Model file for the job. Use its own axes, mm. A direction names the side the tool comes from. Round coordinates to 2 decimals unless told otherwise and drop trailing zeros. Loops run counter-clockwise (first coordinate to the right, second up) from the corner with the lowest first, then second, coordinate; pieces in that order, holes last. Notation, with made-up numbers: (86.25, -18.5) -> (114.25, -18.5) arc R24 ccw to (114.25, -2.5) -> close; hole circle Ø9 at (10, 72). An arc over 180 degrees is marked (long way). Use a Markdown table: item, result. Add a question column.
```python
from build123d import *

# Parameters (mm, degrees)
SKETCH1_R           = 38.1
BOSS_EXTRUDE1_DEPTH = 76.2
SKETCH2_W           = 63.5
SKETCH2_H           = 42.121134838
BOSS_EXTRUDE2_DEPTH = 63.5
SKETCH3_W           = 25.4
SKETCH3_H           = 42.121134838
CUT_EXTRUDE1_DEPTH  = 63.5
FILLET1_R           = 25.4
SKETCH5_R           = 25.4
CUT_EXTRUDE3_DEPTH  = 50.8
SKETCH6_R           = 12.7
BOSS_EXTRUDE3_DEPTH = 53.34


with BuildPart() as part:
    # Sketch1 → Boss-Extrude1 (new body)
    with BuildSketch(Plane(origin=(0, 0, 0), x_dir=(1, 0, 0), z_dir=(0, 1, 0))):
        with Locations(Location((0, 0, 0), (0, 0, 90))):
            Circle(SKETCH1_R)
    extrude(amount=BOSS_EXTRUDE1_DEPTH)

    # Sketch2 → Boss-Extrude2 (add)
    with BuildSketch(Plane(origin=(0, 76.2, 0), x_dir=(1, 0, 0), z_dir=(0, 1, 0))):
        Rectangle(SKETCH2_W, SKETCH2_H)
    extrude(amount=BOSS_EXTRUDE2_DEPTH)

    # Sketch3 → Cut-Extrude1 (cut)
    with BuildSketch(Plane(origin=(0, 139.7, 0), x_dir=(1, 0, 0), z_dir=(0, 1, 0))):
        Rectangle(SKETCH3_W, SKETCH3_H)
    extrude(amount=-CUT_EXTRUDE1_DEPTH, mode=Mode.SUBTRACT)

    # Fillet1
    # the kernel refuses this fillet: 25.4 mm, written as the material it takes off along each edge
    with BuildSketch(Plane(origin=(50.8, 139.7, -21.060567419), x_dir=(0, -1, 0), z_dir=(-1, 0, 0)), Plane(origin=(-95.25, 139.7, 21.060567419), x_dir=(0, -1, 0), z_dir=(1, 0, 0)), Plane(origin=(95.25, 139.7, -21.060567419), x_dir=(0, -1, 0), z_dir=(-1, 0, 0)), Plane(origin=(-50.8, 139.7, 21.060567419), x_dir=(0, -1, 0), z_dir=(1, 0, 0))) as fillet1_piece_1:
        with BuildLine():
            CenterArc((FILLET1_R, FILLET1_R), FILLET1_R, 180, 90)
            Line((0, FILLET1_R), (0, 0))
            Line((0, 0), (FILLET1_R, 0))
        make_face()
    extrude(amount=146.05, mode=Mode.SUBTRACT)

    # Sketch5 → Cut-Extrude3 (cut)
    with BuildSketch(Plane.XZ):
        with Locations(Location((0, 0, 0), (0, 0, 270))):
            Circle(SKETCH5_R)
    extrude(amount=-CUT_EXTRUDE3_DEPTH, mode=Mode.SUBTRACT)

    # Sketch6 → Boss-Extrude3 (add)
    with BuildSketch(Plane(origin=(31.75, 0, 0), x_dir=(0, 0, -1), z_dir=(1, 0, 0))):
        with Locations((0, 114.3)):
            Circle(SKETCH6_R)
    extrude(amount=-BOSS_EXTRUDE3_DEPTH)


solid = part.part
```
1) Pin check, flat tips, straight feed: pin 1 Ø6 at (x, y) = (-16.5, 67) entering from -Z; pin 2 Ø21 at (y, z) = (115, 0) entering from +X; pin 3 Ø7 at (x, z) = (36, -1) entering from +Y. Stop position of each tip, or through.
2) Wall check: probe 1 along X at (y, z) = (93, 13.5); probe 2 along X at (y, z) = (17, 0); probe 3 along Y at (x, z) = (-22.5, -22). Give the ranges that are in metal, low to high. Write a range as from..to.
3) Cut at A-A on x = 0. Write the cut outline in (y, z).
4) Cut at C-C on z = 8. Write the cut outline in (x, y), and give its area (3 significant figures).
5) Pull direction Z, two halves, no side cores. Call faces 1 (the face through (0, 50.8, 0)), 2 (the face through (22.092, 130.844, 14.934)), 3 (the face through (-15.456, 25.044, 20.157)), 4 (the face through (-31.75, 107, 0)): +Z half, -Z half, draft (parallel to the pull), parting line (faces both ways), or undercut.
6) Tool access for faces 5 (the face through (-22, 95, 21.061)), 6 (the face through (22, 95, -21.061)), 7 (the face through (0.18, 101.9, 2.75)), 8 (the face through (31.75, 108, 0)): list every direction of +Z, -Z, +X, -X, +Y, -Y with a clear straight run to the whole face (end or side of a thin tool).
7) Cut at B-B on y = 112. Write the cut outline in (x, z).
8) Cut at D-D on y = 12. Write the cut outline in (x, z), and give its area (3 significant figures).
Established:
| question | item | result |
|---|---|---|
| 1 | pin 1 | stops at z = -35.63 |
| 1 | pin 2 | stops at x = 31.75 |
| 1 | pin 3 | stops at y = 76.2 |
| 2 | probe 1 | x = -31.75..-12.7, 12.7..31.75 |
| 2 | probe 2 | x = -38.1..-25.4, 25.4..38.1 |
| 2 | probe 3 | y = 0..76.2 |
| 3 | outline | (0, -38.1) -> (76.2, -38.1) -> (76.2, 38.1) -> (0, 38.1) -> (0, 25.4) -> (50.8, 25.4) -> (50.8, -25.4) -> (0, -25.4) -> close; circle Ø25.4 at (114.3, 0) |
| 4 | outline | (-37.25, 0) -> (-24.11, 0) -> (-24.11, 50.8) -> (24.11, 50.8) -> (24.11, 0) -> (37.25, 0) -> (37.25, 76.2) -> (31.75, 76.2) -> (31.75, 136.5) -> (12.7, 136.5) -> (12.7, 124.16) -> (-12.7, 124.16) -> (-12.7, 136.5) -> (-31.75, 136.5) -> (-31.75, 76.2) -> (-37.25, 76.2) -> close; hole (-12.7, 76.2) -> (12.7, 76.2) -> (12.7, 104.44) -> (-12.7, 104.44) -> close |
| 4 | area | 6,030 mm^2 |
| 5 | face 1 | undercut |
| 5 | face 2 | +Z half |
| 5 | face 3 | undercut |
| 5 | face 4 | draft |
| 6 | face 5 | +Z, +X, -X, +Y |
| 6 | face 6 | -Z, +X, -X, +Y |
| 6 | face 7 | none |
| 6 | face 8 | +Z, -Z, +X, +Y |
| 7 | outline | (-31.75, -21.06) -> (-12.7, -21.06) -> (-12.7, -12.49) -> (12.7, -12.49) -> (12.7, -21.06) -> (31.75, -21.06) -> (31.75, 21.06) -> (12.7, 21.06) -> (12.7, 12.49) -> (-12.7, 12.49) -> (-12.7, 21.06) -> (-31.75, 21.06) -> close |
| 8 | outline | circle Ø76.2 at (0, 0); hole circle Ø50.8 at (0, 0) |
| 8 | area | 2,530 mm^2 |
